Source: CAD feature listing. Evaluate the final solid. Frame: model axes, mm. Give positions to 0.01 mm unless a question says otherwise; leave off trailing zeros. Order: outer loops, then holes, each group sorted by start corner. A loop starts at its lowest first (then second) coordinate and runs counter-clockwise, first axis right, second up.
from build123d import *

# Parameters (mm, degrees)
ESBO_O1_R                = 2.79
RESSALTO_EXTRUS_O1_DEPTH = 144


with BuildPart() as part:
    # Esboço1 → Ressalto-extrusão1 (new body)
    with BuildSketch(Plane(origin=(0, 85, 0), x_dir=(1, 0, 0), z_dir=(0, 1, 0))):
        with BuildLine():
            Line((6.162658774, -1.825961894), (7.216878365, 0))
            Line((7.216878365, 0), (6.162658774, 1.825961894))
            ThreePointArc((6.162658774, 1.825961894), (4.113620668, 2.375), (4.662658774, 4.424038106))
            Line((4.662658774, 4.424038106), (3.608439182, 6.25))
            Line((3.608439182, 6.25), (1.5, 6.25))
            ThreePointArc((1.5, 6.25), (0, 4.75), (-1.5, 6.25))
            Line((-1.5, 6.25), (-3.608439182, 6.25))
            Line((-3.608439182, 6.25), (-4.662658774, 4.424038106))
            ThreePointArc((-4.662658774, 4.424038106), (-4.113620668, 2.375), (-6.162658774, 1.825961894))
            Line((-6.162658774, 1.825961894), (-7.216878365, 0))
            Line((-7.216878365, 0), (-6.162658774, -1.825961894))
            ThreePointArc((-6.162658774, -1.825961894), (-4.113620668, -2.375), (-4.662658774, -4.424038106))
            Line((-4.662658774, -4.424038106), (-3.608439182, -6.25))
            Line((-3.608439182, -6.25), (-1.5, -6.25))
            ThreePointArc((-1.5, -6.25), (0, -4.75), (1.5, -6.25))
            Line((1.5, -6.25), (3.608439182, -6.25))
            Line((3.608439182, -6.25), (4.662658774, -4.424038106))
            ThreePointArc((4.662658774, -4.424038106), (4.113620668, -2.375), (6.162658774, -1.825961894))
        make_face()
        Circle(ESBO_O1_R, mode=Mode.SUBTRACT)
    extrude(amount=-RESSALTO_EXTRUS_O1_DEPTH)


solid = part.part
1) Pull-direction query (X, two-part tool) for faces 1 (the face through (4.13, 14.01, -2.35)), 2 (the face through (0, -59, -3)); classes: +X half, -X half, draft (parallel to the pull), parting line (faces both ways), or undercut.
Checks:
face 1: undercut
face 2: draft
2) First-contact query: pin 1 Ø1 at (x, y) = (-4.5, 4.5) entering from +Z; pin 2 Ø2 at (y, z) = (55, 2) entering from +X. Flat tips, straight axial feed; report the tip coordinate or a pass-through.
Checks:
pin 1: stops at z = 5.57
pin 2: stops at x = 6.64
3) Section query A-A on y = 27. Output: boundary loops of the cut face in (x, z) (3 decimals), and give its area (3 significant figures).
Checks:
outline: (-7.217, 0) - (-6.163, -1.826) arc R1.5 cw to (-4.663, -4.424) - (-3.608, -6.25) - (-1.5, -6.25) arc R1.5 cw to (1.5, -6.25) - (3.608, -6.25) - (4.663, -4.424) arc R1.5 cw to (6.163, -1.826) - (7.217, 0) - (6.163, 1.826) arc R1.5 cw to (4.663, 4.424) - (3.608, 6.25) - (1.5, 6.25) arc R1.5 cw to (-1.5, 6.25) - (-3.608, 6.25) - (-4.663, 4.424) arc R1.5 cw to (-6.163, 1.826) - close; hole circle Ø5.58 at (0, 0)
area: 89.7 mm2
4) Ray query, L1, parallel to X at y = 19.5, z = 0; L2, parallel to Z at x = 0, y = 28; L3, parallel to X at y = -30, z = -0.5. Return the intervals inside material, ascending.
Checks:
L1: x = -7.22 to -2.79, 2.79 to 7.22
L2: z = -4.75 to -2.79, 2.79 to 4.75
L3: x = -6.93 to -2.74, 2.74 to 6.93
5) Section query B-B on x = 0. Output: boundary loops of the cut face in (y, z), and give its area (3 significant figures).
Checks:
outline: (-59, -4.75) - (85, -4.75) - (85, -2.79) - (-59, -2.79) - close; (-59, 2.79) - (85, 2.79) - (85, 4.75) - (-59, 4.75) - close
area: 564 mm2
